```python
from build123d import *

# Parameters (mm, degrees)
ESQUISSE1_W        = 25.4
ESQUISSE1_H        = 40.8
ESQUISSE1_R        = 1.75
ESQUISSE1_R_2      = 1.816105755
BOSS_EXTRU_1_DEPTH = 1.6
ESQUISSE2_W        = 10
ESQUISSE2_H        = 10.5
BOSS_EXTRU_2_DEPTH = 2.4
ESQUISSE3_R        = 1.75
BOSS_EXTRU_3_DEPTH = 7.1


with BuildPart() as part:
    # Esquisse1 → Boss.-Extru.1 (new body)
    with BuildSketch(Plane.XY):
        with Locations((54.255448742, 40.424731349)):
            Rectangle(ESQUISSE1_W, ESQUISSE1_H)
        with Locations((62.755448742, 25.479221209)):
            Circle(ESQUISSE1_R, mode=Mode.SUBTRACT)
        with Locations((45.755448742, 25.479221209)):
            Circle(ESQUISSE1_R, mode=Mode.SUBTRACT)
        with Locations((62.755448742, 48.479221209)):
            Circle(ESQUISSE1_R, mode=Mode.SUBTRACT)
        with Locations((45.755448742, 48.479221209)):
            Circle(ESQUISSE1_R, mode=Mode.SUBTRACT)
        with Locations((54.255448742, 39.024731349)):
            Circle(ESQUISSE1_R_2, mode=Mode.SUBTRACT)
    extrude(amount=BOSS_EXTRU_1_DEPTH)

    # Esquisse2 → Boss.-Extru.2 (add)
    with BuildSketch(Plane.XY.offset(1.6)):
        with Locations((54.255448742, 39.024731349)):
            Rectangle(ESQUISSE2_W, ESQUISSE2_H)
    extrude(amount=BOSS_EXTRU_2_DEPTH)

    # Esquisse3 → Boss.-Extru.3 (add)
    with BuildSketch(Plane.XY.offset(4)):
        with Locations((54.255448742, 39.024731349)):
            Circle(ESQUISSE3_R)
    extrude(amount=BOSS_EXTRU_3_DEPTH)


solid = part.part
```
Design review of the part built by this model. Coordinates are the model's own, in mm. A direction names the side the tool comes from. Coordinates: 2 decimals unless noted, no trailing zeros. Loops run counter-clockwise (first coordinate to the right, second up) from the corner with the lowest first, then second, coordinate; pieces in that order, holes last.
Q1. We need section D-D on y = 24.5. State the section outline as (x, z) points.
Reported:
outline: (41.56, 0) - (44.31, 0) - (44.31, 1.6) - (41.56, 1.6) - close; (47.21, 0) - (61.31, 0) - (61.31, 1.6) - (47.21, 1.6) - close; (64.21, 0) - (66.96, 0) - (66.96, 1.6) - (64.21, 1.6) - close
Q2. For pin 1 (1.1 mm diameter, centred on x = 54, y = 38.5, fed in from -Z); pin 2 (2 mm diameter, centred on x = 45.76, y = 25.48, fed in from -Z); pin 3 (4 mm diameter, centred on x = 58.5, y = 49, fed in from +Z); pin 4 (4 mm diameter, centred on y = 40.5, z = 6.5, fed in from +X), all flat-tipped, find the tip position at first contact; note any pin that passes through.
Reported:
pin 1: stops at z = 1.6
pin 2: passes through
pin 3: stops at z = 1.6
pin 4: stops at x = 56.01
Q3. To check wall thickness, follow line 1 (X direction, y = 39, z = 4.25); line 2 (Z direction, x = 47.75, y = 53); line 3 (X direction, y = 37.5, z = 3). State the ranges of each line that lie inside material, in increasing order.
Reported:
line 1: x = 52.51 to 56.01
line 2: z = 0 to 1.6
line 3: x = 49.26 to 59.26
Q4. We need section C-C on x = 46.5. State the section outline as (y, z) points.
Reported:
outline: (20.02, 0) - (23.9, 0) - (23.9, 1.6) - (20.02, 1.6) - close; (27.06, 0) - (46.9, 0) - (46.9, 1.6) - (27.06, 1.6) - close; (50.06, 0) - (60.82, 0) - (60.82, 1.6) - (50.06, 1.6) - close
Q5. Tool access review of faces 1 (the face through (59.255, 39, 3)), 2 (the face through (55.988, 39.57, 0.789)), 3 (the face through (56.4, 39.1, 4)), 4 (the face through (54, 44.275, 3)), 5 (the face through (54, 33.775, 3)): name each direction out of +Z, -Z, +X, -X, +Y, -Y from which nothing blocks a thin tool from reaching the whole face with its end or side.
Reported:
face 1: +Z, +X, +Y, -Y
face 2: -Z
face 3: +Z
face 4: +Z, +X, -X, +Y
face 5: +Z, +X, -X, -Y
Q6. We need section A-A on x = 57.25. State the section outline as (y, z) points.
Reported:
outline: (20.02, 0) - (60.82, 0) - (60.82, 1.6) - (44.27, 1.6) - (44.27, 4) - (33.77, 4) - (33.77, 1.6) - (20.02, 1.6) - close
Q7. The part is to be moulded in two halves that separate along Y. For faces 6 (the face through (47.372, 24.809, 0.789)), 7 (the face through (49.255, 39, 3)), 8 (the face through (52.867, 37.96, 7.5)), say which applies: +Y half, -Y half, draft (parallel to the pull), parting line (faces both ways), or undercut.
Reported:
face 6: undercut
face 7: draft
face 8: parting line
Q8. We need section B-B on z = 0.75. State the section outline as (x, y) points, and give its area (3 significant figures).
Reported:
outline: (41.56, 20.02) - (66.96, 20.02) - (66.96, 60.82) - (41.56, 60.82) - close; hole circle Ø3.5 at (45.76, 25.48); hole circle Ø3.5 at (45.76, 48.48); hole circle Ø3.63 at (54.26, 39.02); hole circle Ø3.5 at (62.76, 25.48); hole circle Ø3.5 at (62.76, 48.48)
area: 987 mm2
